Geometry check sheet. Reference: the model listing, model coordinates, mm. Face numbers are marked on the shaded views. Round coordinates to 2 decimals unless told otherwise and drop trailing zeros. Write each loop counter-clockwise with the first axis right and the second up, starting at its lowest first coordinate (ties: lowest second). Pieces come first, ordered by that corner, then holes. Notation, with made-up numbers: M 56.5,18.25 L 112.5,18.25 A29 cw 112.5,38.25 Z; hole C -32,13.25 d1. An arc over 180 degrees is marked long. Put each result on its own line as item: value. Start each with the question number.
(1) Material ranges on probe 1 along Z at (x, y) = (-46, 29); probe 2 along Y at (x, z) = (0, 94) (3 decimals), recorded low to high.
(2) Mould release check, pull along X, two halves, no side actions. Record for the marked faces 1 and 2: pulls with the +X half, pulls with the -X half, needs draft (parallel to the pull), parting line crosses it, or undercut.
(3) Gauge pin test, flat ends, axial feed: pin 1 (5 mm diameter, centred on y = -41.5, z = 184.5, fed in from -X); pin 2 (1.5 mm diameter, centred on x = 21, z = 237.5, fed in from +Y); pin 3 (2 mm diameter, centred on x = -17.5, z = 113.5, fed in from -Y). Record the tip position at first contact, or that the pin passes through.
(4) Section check C-C on z = 136. Record the cut outline in (x, y) (3 decimals).
(5) Section check D-D on y = -21.5. Record the cut outline in (x, z).
(6) Section check A-A on x = 0. Record the cut outline in (y, z) (3 decimals), then the cut area to 3 significant figures.
from build123d import *

# Parameters (mm, degrees)
SKETCH1_R      = 57.15
SKETCH1_R_2    = 53.975
EXTRUDE1_DEPTH = 304.8
SKETCH2_W      = 76.2
SKETCH2_H      = 203.2
EXTRUDE2_DEPTH = 316.333609056
SKETCH3_W      = 203.2
SKETCH3_H      = 76.2
EXTRUDE3_DEPTH = 316.333609056


with BuildPart() as part:
    # Sketch1 → Extrude1 (new body)
    with BuildSketch(Plane.XY):
        with Locations(Location((0, 0, 0), (0, 0, 180))):
            Circle(SKETCH1_R)
        with Locations(Location((0, 0, 0), (0, 0, 180))):
            Circle(SKETCH1_R_2, mode=Mode.SUBTRACT)
    extrude(amount=EXTRUDE1_DEPTH)

    # Sketch2 → Extrude2 (cut, through all)
    with BuildSketch(Plane(origin=(0, 0, 0), x_dir=(1, 0, 0), z_dir=(0, 1, 0))):
        with Locations((0, -152.4)):
            Rectangle(SKETCH2_W, SKETCH2_H)
    extrude(amount=-EXTRUDE2_DEPTH, mode=Mode.SUBTRACT)

    # Sketch3 → Extrude3 (cut, through all)
    with BuildSketch(Plane(origin=(0, 0, 0), x_dir=(0, 0, -1), z_dir=(0.8660254037844365, -0.500000000000004, 0))):
        with Locations((-152.4, 0)):
            Rectangle(SKETCH3_W, SKETCH3_H)
    extrude(amount=-EXTRUDE3_DEPTH, mode=Mode.SUBTRACT)


solid = part.part
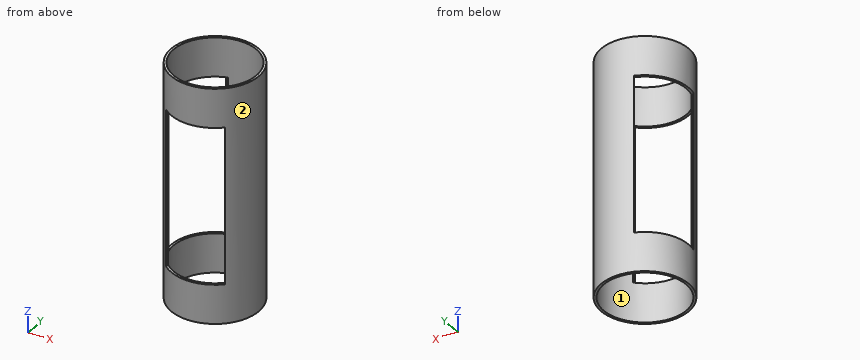
Answers follow:
1. probe 1: z = 0 to 50.8, 254 to 304.8
1. probe 2: y = 53.975 to 57.15
2. face 1: undercut
2. face 2: parting line crosses it
3. pin 1: stops at x = -41.77
3. pin 2: stops at y = 53.44
3. pin 3: stops at y = 53.52
4. outline: M -55.94,-11.697 A57.15 ccw -38.1,-42.597 L -38.1,-38.232 A53.975 cw -52.16,-13.88 Z; M -17.84,54.294 L -14.06,52.112 A53.975 cw 38.1,-38.232 L 38.1,-42.597 A57.15 ccw Z
5. outline: M -52.95,0 L -49.51,0 L -49.51,304.8 L -52.95,304.8 Z; M 49.51,0 L 52.95,0 L 52.95,304.8 L 49.51,304.8 Z
6. outline: M -57.15,0 L -53.975,0 L -53.975,50.8 L -57.15,50.8 Z; M -57.15,254 L -53.975,254 L -53.975,304.8 L -57.15,304.8 Z; M 53.975,0 L 57.15,0 L 57.15,304.8 L 53.975,304.8 Z
6. area: 1,290 mm^2
